Autodesk Inventor part; units mm, degrees
ref_plane "YZ Plane" through (0, 0, 0) normal (1, 0, 0) x (0, 1, 0)
ref_plane "XZ Plane" through (0, 0, 0) normal (0, 1, 0) x (-1, 0, 0)
ref_plane "XY Plane" through (0, 0, 0) normal (0, 0, 1) x (1, 0, 0)
sketch "Sketch1" plane through (0, 0, 0) normal (0, 1, 0) x (-1, 0, 0)
  point P0 (0, 0)
sketch "Sketch2" plane through (0, 0, 0) normal (0, 1, 0) x (-1, 0, 0)
  line L0 (-100, 100) -> (100, 100)
  line L1 (100, 100) -> (100, -100)
  line L2 (100, -100) -> (-100, -100)
  line L3 (-100, -100) -> (-100, 100)
  line L4 (-100, 100) -> (100, -100) construction
  line L5 (100, 100) -> (-100, -100) construction
  line L6 (27, -18.5) -> (33, -18.5)
  line L7 (33, -18.5) -> (33, -6.5)
  line L8 (33, -6.5) -> (27, -6.5)
  line L9 (27, -6.5) -> (27, -18.5)
  line L10 (27, -18.5) -> (33, -6.5) construction
  line L11 (33, -18.5) -> (27, -6.5) construction
  line L12 (0, 100) -> (0, -100) construction
  line L13 (100, 0) -> (-100, 0) construction
  circle A0 centre (0, 0) radius 5
  circle A1 centre (16, -16) radius 4.5
  circle A2 centre (-16, 16) radius 4.5
  line L14 (8, -13.5) -> (-22, -13.5)
  line L15 (-22, -13.5) -> (-22, -18.5)
  line L16 (-22, -18.5) -> (8, -18.5)
  line L17 (8, -18.5) -> (8, -13.5)
  line L18 (-8, 13.5) -> (22, 13.5)
  line L19 (22, 13.5) -> (22, 18.5)
  line L20 (22, 18.5) -> (-8, 18.5)
  line L21 (-8, 18.5) -> (-8, 13.5)
  circle A3 centre (18.9997, 0) radius 1
  circle A4 centre (-18.9997, 0) radius 1
  line L22 (27, 18.5) -> (33, 18.5)
  line L23 (33, 18.5) -> (33, 6.5)
  line L24 (33, 6.5) -> (27, 6.5)
  line L25 (27, 6.5) -> (27, 18.5)
  line L26 (27, 18.5) -> (33, 6.5) construction
  line L27 (33, 18.5) -> (27, 6.5) construction
  line L28 (-27, -18.5) -> (-33, -18.5)
  line L29 (-33, -18.5) -> (-33, -6.5)
  line L30 (-33, -6.5) -> (-27, -6.5)
  line L31 (-27, -6.5) -> (-27, -18.5)
  line L32 (-27, -18.5) -> (-33, -6.5) construction
  line L33 (-33, -18.5) -> (-27, -6.5) construction
  line L34 (-27, 6.5) -> (-27, 18.5)
  line L35 (-27, 18.5) -> (-33, 18.5)
  line L36 (-33, 18.5) -> (-33, 6.5)
  line L37 (-27, 18.5) -> (-33, 6.5) construction
  line L38 (-33, 18.5) -> (-27, 6.5) construction
  line L39 (-33, 6.5) -> (-27, 6.5)
  circle A5 centre (16, 16) radius 4.5
  circle A6 centre (-16, -16) radius 4.5
  point P0 (30, -12.5)
  point P1 (30, 12.5)
  point P2 (-30, -12.5)
  point P3 (-30, 12.5)
  dimension "d0" = 200
  dimension "d1" = 200
  dimension "d3" = 12
  dimension "d5" = 10
  dimension "d8" = 9
  dimension "d10" = 16
  dimension "d11" = 16
  dimension "d15" = 30
  dimension "d16" = 5
  dimension "d17" = 13.5
  dimension "d18" = 8
  dimension "d19" = 30
  dimension "d20" = 5
  dimension "d21" = 13.5
  dimension "d22" = 8
  dimension "d23" = 2
  dimension "d24" = 8.0003
  dimension "d27" = 6
  dimension "d30" = 30
extrude "Extrusion1" add sketch "Sketch2" along normal blind 6
properties part number "thumper-base-v2"
The model under review builds one solid part; all positions refer to its coordinate system, in mm. A direction names the side the tool comes from. Round coordinates to 2 decimals unless told otherwise and drop trailing zeros. Write each loop counter-clockwise with the first axis right and the second up, starting at its lowest first coordinate (ties: lowest second). Pieces come first, ordered by that corner, then holes. Notation, with made-up numbers: M -10.75,-7.5 L 13.25,-7.5 A29 ccw 13.25,12.5 Z; hole C -8,63 d8. An arc over 180 degrees is marked long. Use CSV: the item, a comma, the result in double quotes. Start each with the question number.
(1) For line 1 along Z through (x, y) = (-16, 3.85); line 2 along X through (y, z) = (4.45, 9); line 3 along Z through (x, y) = (29.5, 3), list the stretches that pass through material, from the lowest coordinate up.
(2) We need section B-B, the plane x = 0. State the section outline as (y, z) points, then the cut area to 3 significant figures.
(3) We need section C-C, the plane y = 3.6. State how many separate pieces and enclosed holes the cut face has, then the cut area to 3 significant figures.
(4) We need section A-A, the plane z = 16. State the section outline as (x, y) points, then the cut area to 3 significant figures.
(5) The part is to be moulded in two halves that separate along X. For faces 3 (the face through (-30, 3, 18.5)), 4 (the face through (-100, 3, 1)), 5 (the face through (1, 3, 100)), say which applies: +X half, -X half, draft (parallel to the pull), parting line (faces both ways), or undercut.
(6) Tool access review of faces 1 (the face through (-1, 3, -100)), 2 (the face through (2, 3, -13.5)): name each direction out of +Z, -Z, +X, -X, +Y, -Y from which nothing blocks a thin tool from reaching the whole face with its end or side.
Findings:
1,line 1,"-100 to -20.5, -11.5 to 11.5, 20.5 to 100"
1,line 2,"-100 to -33, -27 to 27, 33 to 100"
1,line 3,"-100 to -18.5, -6.5 to 6.5, 18.5 to 100"
2,outline,"M 0,-100 L 6,-100 L 6,-18.5 L 0,-18.5 Z; M 0,-13.5 L 6,-13.5 L 6,-5 L 0,-5 Z; M 0,5 L 6,5 L 6,13.5 L 0,13.5 Z; M 0,18.5 L 6,18.5 L 6,100 L 0,100 Z"
2,area,"1,080 mm^2"
3,separate pieces,"1"
3,enclosed holes,"11"
3,area,"39,200 mm^2"
4,outline,"M -100,0 L -33,0 L -33,6 L -100,6 Z; M -27,0 L -22,0 L -22,6 L -27,6 Z; M 8,0 L 11.5,0 L 11.5,6 L 8,6 Z; M 20.5,0 L 27,0 L 27,6 L 20.5,6 Z; M 33,0 L 100,0 L 100,6 L 33,6 Z"
4,area,"894 mm^2"
5,face 3,"undercut"
5,face 4,"-X half"
5,face 5,"draft"
6,face 1,"-Z, +X, -X, +Y, -Y"
6,face 2,"+Y, -Y"
